Check sheet for the modelled part. Datum: model origin and axes. Units: mm. A direction names the side the tool comes from. Coordinates: 2 decimals unless noted, no trailing zeros. Write each loop counter-clockwise with the first axis right and the second up, starting at its lowest first coordinate (ties: lowest second). Pieces come first, ordered by that corner, then holes. Notation, with made-up numbers: (14.5, -0.75) -> (50.5, -0.75) arc R11 ccw to (50.5, 3.25) -> close; hole circle Ø4 at (-28.75, 35). An arc over 180 degrees is marked (long way). Put each result on its own line as item: value.
```python
from build123d import *

# Parameters (mm, degrees)
SKETCH_1_W          = 145
SKETCH_1_H          = 61.5
SKETCH_1_R          = 2
EXTRUDE_1_DEPTH     = 3
SKETCH_2_R          = 2
CUT_EXTRUDE_1_DEPTH = 10
SKETCH_3_R          = 1.5
CUT_EXTRUDE_2_DEPTH = 10
FILLET_2_R          = 2


with BuildPart() as part:
    # 草图1 → 凸台-拉伸1 (new body)
    with BuildSketch(Plane(origin=(0, 0, 0), x_dir=(1, 0, 0), z_dir=(0, 1, 0))):
        with Locations((0, -8.25)):
            Rectangle(SKETCH_1_W, SKETCH_1_H)
        with Locations(Location((-67.5, 12.5, 0), (0, 0, 270))):
            Circle(SKETCH_1_R, mode=Mode.SUBTRACT)
        with Locations(Location((-67.5, -12.5, 0), (0, 0, 270))):
            Circle(SKETCH_1_R, mode=Mode.SUBTRACT)
        with Locations(Location((67.5, 12.5, 0), (0, 0, 270))):
            Circle(SKETCH_1_R, mode=Mode.SUBTRACT)
        with Locations(Location((67.5, -12.5, 0), (0, 0, 270))):
            Circle(SKETCH_1_R, mode=Mode.SUBTRACT)
        with Locations(Location((15, 12.5, 0), (0, 0, 270))):
            Circle(SKETCH_1_R, mode=Mode.SUBTRACT)
        with Locations(Location((15, -12.5, 0), (0, 0, 270))):
            Circle(SKETCH_1_R, mode=Mode.SUBTRACT)
        with Locations(Location((-47.5, 12.5, 0), (0, 0, 270))):
            Circle(SKETCH_1_R, mode=Mode.SUBTRACT)
        with Locations(Location((-47.5, -12.5, 0), (0, 0, 270))):
            Circle(SKETCH_1_R, mode=Mode.SUBTRACT)
        with Locations(Location((47.5, 12.5, 0), (0, 0, 270))):
            Circle(SKETCH_1_R, mode=Mode.SUBTRACT)
        with Locations(Location((47.5, -12.5, 0), (0, 0, 270))):
            Circle(SKETCH_1_R, mode=Mode.SUBTRACT)
    extrude(amount=EXTRUDE_1_DEPTH)

    # 草图2 → 切除-拉伸1 (cut)
    with BuildSketch(Plane(origin=(0, 3, 0), x_dir=(1, 0, 0), z_dir=(0, 1, 0))):
        with Locations(Location((-12.5, -4, 0), (0, 0, 270))):
            Circle(SKETCH_2_R)
        with Locations(Location((12.5, -4, 0), (0, 0, 270))):
            Circle(SKETCH_2_R)
        Polygon((-52.5, -39), (-52.5, -24), (-20, -24), (-20, -9), (20, -9), (20, -24), (52.5, -24), (52.5, -39), align=None)
    extrude(amount=-CUT_EXTRUDE_1_DEPTH, mode=Mode.SUBTRACT)

    # 草图3 → 切除-拉伸2 (cut)
    with BuildSketch(Plane(origin=(0, 3, 0), x_dir=(1, 0, 0), z_dir=(0, 1, 0))):
        with Locations((-47.5, 12.5)):
            Circle(SKETCH_3_R)
        with Locations(Location((-47.5, -7.5, 0), (0, 0, 270))):
            Circle(SKETCH_3_R)
        with Locations(Location((31.3, 12.5, 0), (0, 0, 270))):
            Circle(SKETCH_3_R)
        with Locations(Location((31.3, -7.5, 0), (0, 0, 270))):
            Circle(SKETCH_3_R)
        with Locations(Location((-28.6, 12.5, 0), (0, 0, 270))):
            Circle(SKETCH_3_R)
        with Locations(Location((-28.6, -7.5, 0), (0, 0, 270))):
            Circle(SKETCH_3_R)
    extrude(amount=-CUT_EXTRUDE_2_DEPTH, mode=Mode.SUBTRACT)

    # 圆角2
    fillet_2_edges = [part.edges().sort_by_distance(p)[0] for p in [
        (52.5, 1.5, 39),
        (-52.5, 1.5, 39),
        (-52.5, 1.5, 24),
        (-20, 1.5, 24),
        (-20, 1.5, 9),
        (20, 1.5, 9),
        (20, 1.5, 24),
        (52.5, 1.5, 24),
        (72.5, 1.5, -22.5),
        (72.5, 1.5, 39),
        (-72.5, 1.5, 39),
        (-72.5, 1.5, -22.5),
    ]]
    fillet(fillet_2_edges, radius=FILLET_2_R)


solid = part.part
```
Q1. Cross-section at B-B (z = 4). Record the cut outline in (x, y), plus the area to 3 significant figures.
Recorded:
outline: (-72.5, 0) -> (-14.5, 0) -> (-14.5, 3) -> (-72.5, 3) -> close; (-10.5, 0) -> (10.5, 0) -> (10.5, 3) -> (-10.5, 3) -> close; (14.5, 0) -> (72.5, 0) -> (72.5, 3) -> (14.5, 3) -> close
area: 411 mm2
Q2. Material ranges on line 1 along X through (y, z) = (1.1, 12.5); line 2 along X through (y, z) = (0.65, 7.5); line 3 along X through (y, z) = (2.65, 16), recorded low to high.
Recorded:
line 1: x = -72.5 to -69.5, -65.5 to -49.5, -45.5 to -20, 20 to 45.5, 49.5 to 65.5, 69.5 to 72.5
line 2: x = -72.5 to -49, -46 to -30.1, -27.1 to 29.8, 32.8 to 72.5
line 3: x = -72.5 to -20, 20 to 72.5
Q3. Tool access check on faces 4 (the flat face through (0, 2, 9)), 5 (the cylindrical face through (-65.517, 1.479, 12.24)). Record the directions out of +Z, -Z, +X, -X, +Y, -Y that give a thin tool (end or side, any length) a straight path to the whole face; none if there is none.
Recorded:
face 4: +Z, +Y, -Y
face 5: +Y, -Y
Q4. Depth check by flat-ended pin: P1, Ø3, axis at x = 67.5, z = 12.5, coming from the +Y side; P2, Ø3.5, axis at x = -28.6, z = -12.5, coming from the +Y side; P3, Ø1.5, axis at x = -6, y = 1, coming from the +Z side; P4, Ø1.5, axis at x = -42.5, y = 2, coming from the +Z side. Enter the tip coordinate at first touch or a pass-through.
Recorded:
P1: passes through
P2: stops at y = 3
P3: stops at z = 9
P4: stops at z = 24
Q5. Mould release check, pull along X, two halves, no side actions. Record for faces 1 (the cylindrical face through (69.483, 1.479, -12.76)), 2 (the flat face through (62, 1, 39)), 3 (the flat face through (-72.5, 1, 9)): released by +X, released by -X, zero draft, split by the parting line, or undercut.
Recorded:
face 1: undercut
face 2: zero draft
face 3: released by -X
Q6. Cross-section at D-D (z = 12.5). Record the cut outline in (x, y), plus the area to 3 significant figures.
Recorded:
outline: (-72.5, 0) -> (-69.5, 0) -> (-69.5, 3) -> (-72.5, 3) -> close; (-65.5, 0) -> (-49.5, 0) -> (-49.5, 3) -> (-65.5, 3) -> close; (-45.5, 0) -> (-20, 0) -> (-20, 3) -> (-45.5, 3) -> close; (20, 0) -> (45.5, 0) -> (45.5, 3) -> (20, 3) -> close; (49.5, 0) -> (65.5, 0) -> (65.5, 3) -> (49.5, 3) -> close; (69.5, 0) -> (72.5, 0) -> (72.5, 3) -> (69.5, 3) -> close
area: 267 mm2
Q7. Cross-section at C-C (x = -47.5). Record the cut outline in (y, z), plus the area to 4 significant figures.
Recorded:
outline: (0, -22.5) -> (3, -22.5) -> (3, -14.5) -> (0, -14.5) -> close; (0, -10.5) -> (3, -10.5) -> (3, 6) -> (0, 6) -> close; (0, 9) -> (3, 9) -> (3, 10.5) -> (0, 10.5) -> close; (0, 14.5) -> (3, 14.5) -> (3, 24) -> (0, 24) -> close
area: 106.5 mm2
Q8. Cross-section at A-A (x = 67.5). Record the cut outline in (y, z), plus the area to 4 significant figures.
Recorded:
outline: (0, -22.5) -> (3, -22.5) -> (3, -14.5) -> (0, -14.5) -> close; (0, -10.5) -> (3, -10.5) -> (3, 10.5) -> (0, 10.5) -> close; (0, 14.5) -> (3, 14.5) -> (3, 39) -> (0, 39) -> close
area: 160.5 mm2
